Check sheet for the drawn part. Datum: minimum x, y, z corner. Units: mm. Give positions to 0.01 mm unless a question says otherwise; leave off trailing zeros. Write each loop counter-clockwise with the first axis right and the second up, starting at its lowest first coordinate (ties: lowest second). Pieces come first, ordered by that corner, then holes. Notation, with made-up numbers: (15, -15.75) -> (56, -15.75) arc R6 cw to (56, -8.75) -> close; hole circle Ø3 at (68, 20). An arc over 180 degrees is marked (long way). Write item = value, one per line. Start each with the question number.
1. Cross-section at B-B, the plane x = 3.1. Record the cut outline in (y, z) (3 decimals), plus the area to 3 significant figures.
2. Cross-section at A-A, the plane y = 12.5. Record the cut outline in (x, z) (3 decimals).
3. Cross-section at C-C, the plane y = 20.5. Record the cut outline in (x, z) (3 decimals), plus the area to 3 significant figures.
4. Cross-section at D-D, the plane z = 20. Record the cut outline in (x, y), plus the area to 3 significant figures.
5. Thickness scan on line 1 along Y through (x, z) = (3.3, 58); line 2 along Y through (x, z) = (3.95, 20); line 3 along Z through (x, y) = (4.1, 5.5) (3 decimals). Record the ranges inside material, lowest first.
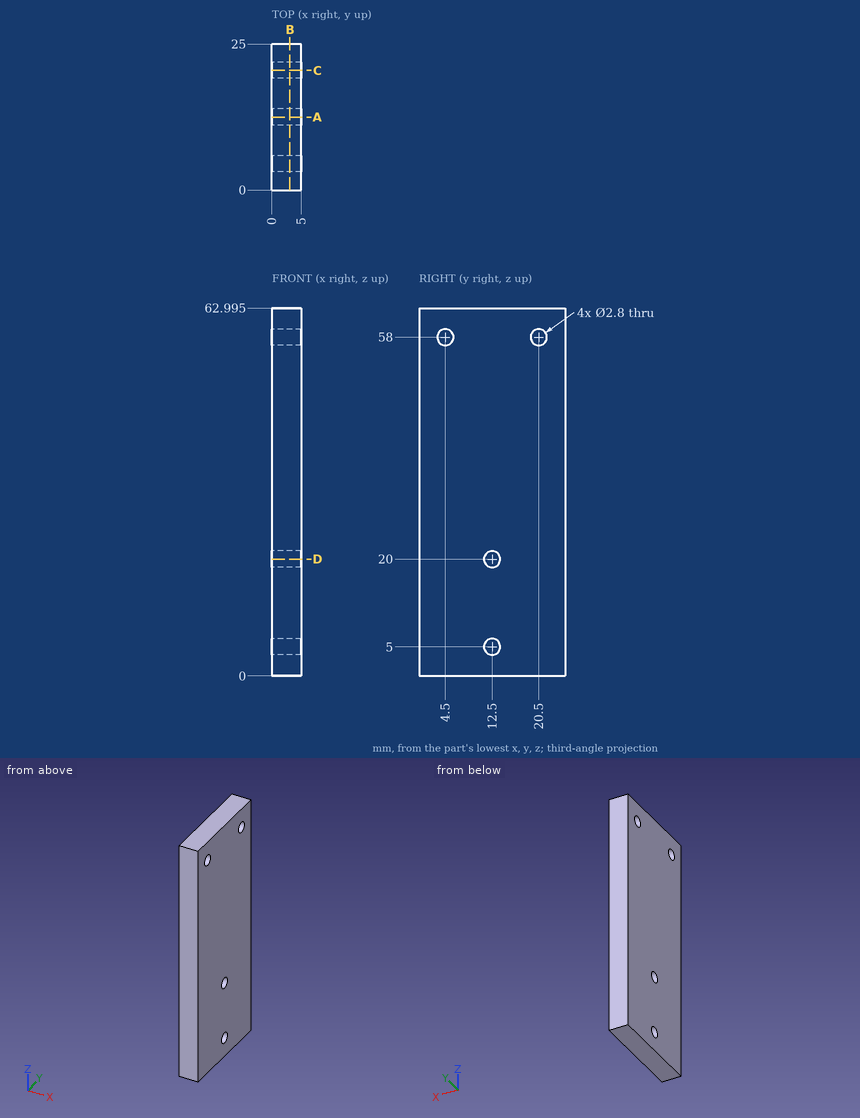
Answers:
q1.outline = (0, 0) -> (25, 0) -> (25, 62.995) -> (0, 62.995) -> close; hole circle Ø2.8 at (4.5, 58); hole circle Ø2.8 at (12.5, 5); hole circle Ø2.8 at (12.5, 20); hole circle Ø2.8 at (20.5, 58)
q1.area = 1,550 mm^2
q2.outline = (0, 0) -> (5, 0) -> (5, 3.6) -> (0, 3.6) -> close; (0, 6.4) -> (5, 6.4) -> (5, 18.6) -> (0, 18.6) -> close; (0, 21.4) -> (5, 21.4) -> (5, 62.995) -> (0, 62.995) -> close
q3.outline = (0, 0) -> (5, 0) -> (5, 56.6) -> (0, 56.6) -> close; (0, 59.4) -> (5, 59.4) -> (5, 62.995) -> (0, 62.995) -> close
q3.area = 301 mm^2
q4.outline = (0, 0) -> (5, 0) -> (5, 11.1) -> (0, 11.1) -> close; (0, 13.9) -> (5, 13.9) -> (5, 25) -> (0, 25) -> close
q4.area = 111 mm^2
q5.line_1 = 0 to 3.1, 5.9 to 19.1, 21.9 to 25
q5.line_2 = 0 to 11.1, 13.9 to 25
q5.line_3 = 0 to 57.02, 58.98 to 62.995
